from build123d import *

# Parameters (mm, degrees)
F0_R     = 2.15
F1_DEPTH = 3.2
F3_DEPTH = 12.5


with BuildPart() as f1:
    # F0 (on Top) → F1 (new body)
    with BuildSketch(Plane.XY):
        with BuildLine():
            ThreePointArc((-8, 50), (-4, 46), (0, 50))
            ThreePointArc((0, 50), (-4, 54), (-8, 50))
        make_face()
        with Locations((-4, 50)):
            Circle(F0_R, mode=Mode.SUBTRACT)
        with BuildLine():
            Line((0, -50), (0, 50))
            ThreePointArc((0, 50), (-4, 46), (-8, 50))
            Line((-8, 50), (-8, -50))
            ThreePointArc((-8, -50), (-4, -46), (0, -50))
        make_face()
        with BuildLine():
            ThreePointArc((-8, -50), (-4, -54), (0, -50))
            ThreePointArc((0, -50), (-4, -46), (-8, -50))
        make_face()
        with Locations((-4, -50)):
            Circle(F0_R, mode=Mode.SUBTRACT)
    extrude(amount=F1_DEPTH)

    # F2 (on Top) → F3 (cut, symmetric)
    with BuildSketch(Plane.XY):
        Polygon((-6.5, -23), (-8, -22), (-8, -29), (-6.5, -28), align=None)
    extrude(amount=F3_DEPTH, both=True, mode=Mode.SUBTRACT)


solid = f1.part
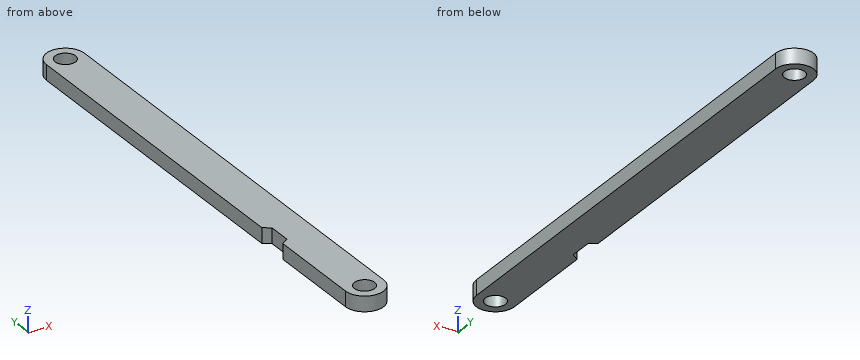
Source: CAD feature listing. Evaluate the final solid. Frame: model axes, mm. Give positions to 0.01 mm unless a question says otherwise; leave off trailing zeros. Write each loop counter-clockwise with the first axis right and the second up, starting at its lowest first coordinate (ties: lowest second). Pieces come first, ordered by that corner, then holes. Notation, with made-up numbers: (-35, 66) - (9, 66) arc R17 ccw to (9, 88) - close; hole circle Ø1 at (28.5, -9). An arc over 180 degrees is marked (long way). Write item = value, one per line. Start each with the question number.
Q1. Material intervals for probe 1 along Y at (x, z) = (-4, 1.2); probe 2 along Y at (x, z) = (-5, 1.85); probe 3 along Y at (x, z) = (-6.75, 1.7), sorted ascending.
Q2. Cut plane A-A, the plane x = -4. Return loops of the section in (y, z), then the cut area to 3 significant figures.
Q3. Pin query (flat end, axial travel): pin 1 Ø1.6 at (y, z) = (-25.5, 1) entering from -X; pin 2 Ø2.5 at (x, y) = (-4, -50) entering from -Z. Return the tip coordinate at first contact, or that it passes through.
Q4. Cut plane B-B, the plane z = 1.2. Return loops of the section in (x, y), then the cut area to 3 significant figures.
Computed values:
q1.probe_1 = -54 to -52.15, -47.85 to 47.85, 52.15 to 54
q1.probe_2 = -53.87 to -51.9, -48.1 to 48.1, 51.9 to 53.87
q1.probe_3 = -52.9 to -28.17, -22.83 to 52.9
q2.outline = (-54, 0) - (-52.15, 0) - (-52.15, 3.2) - (-54, 3.2) - close; (-47.85, 0) - (47.85, 0) - (47.85, 3.2) - (-47.85, 3.2) - close; (52.15, 0) - (54, 0) - (54, 3.2) - (52.15, 3.2) - close
q2.area = 318 mm²
q3.pin_1 = -6.5
q3.pin_2 = through
q4.outline = (-8, -50) arc R4 ccw to (0, -50) - (0, 50) arc R4 ccw to (-8, 50) - (-8, -22) - (-6.5, -23) - (-6.5, -28) - (-8, -29) - close; hole circle Ø4.3 at (-4, -50); hole circle Ø4.3 at (-4, 50)
q4.area = 812 mm²
